```python
from build123d import *

# Parameters (mm, degrees)
F0_W     = 44.45
F0_H     = 44.45
F1_DEPTH = 565.15
F3_DEPTH = 44.45
F5_DEPTH = 44.451
F6_W     = 19.05
F6_H     = 19.05
F7_DEPTH = 19.05


with BuildPart() as f1:
    # F0 (on Top) → F1 (new body)
    with BuildSketch(Plane.XY):
        with Locations((-22.225, 22.225)):
            Rectangle(F0_W, F0_H)
    extrude(amount=-F1_DEPTH)

    # F2 (on face) → F3 (cut, through all)
    with BuildSketch(Plane.XZ):
        Polygon((-9.525, -565.15), (0, -565.15), (0, -488.95), align=None)
    extrude(amount=-F3_DEPTH, mode=Mode.SUBTRACT)

    # F4 (on face) → F5 (cut, through all)
    with BuildSketch(Plane(origin=(-44.45, 0, 0), x_dir=(0, -1, 0), z_dir=(-1, 0, 0))):
        Polygon((0, -565.15), (0, -488.95), (-9.525, -565.15), align=None)
    extrude(amount=-F5_DEPTH, mode=Mode.SUBTRACT)

    # F6 (on face) → F7 (cut)
    with BuildSketch(Plane.XZ):
        with Locations((-9.525, -454.025)):
            Rectangle(F6_W, F6_H)
    extrude(amount=-F7_DEPTH, mode=Mode.SUBTRACT)


solid = f1.part
```
The listing builds one solid part. Answer for the finished solid, in the listing's coordinates (mm). A direction names the side the tool comes from. Give positions to 0.01 mm unless a question says otherwise; leave off trailing zeros.
1) For faces 4 (the face through (-22.536, 4.696, -526.517)), 5 (the face through (-10, 19.05, -454)), determine the directions among +Z, -Z, +X, -X, +Y, -Y from which every point of the face is accessible in a straight line to the end or side of a thin tool.
Reported:
face 4: -Z, +X, -X, -Y
face 5: +X, -Y
2) Determine the mould class of faces 1 (the face through (-4.696, 21.914, -526.517)), 2 (the face through (-10, 9, -444.5)), 3 (the face through (-23, 0, -241)) for opening direction Z: pulls with the +Z half, pulls with the -Z half, needs draft (parallel to the pull), parting line crosses it, or undercut.
Reported:
face 1: pulls with the -Z half
face 2: undercut
face 3: needs draft
3) Consider line 1 along Z through (x, y) = (-14, 16.5); line 2 along X through (y, z) = (22, -498.5); line 3 along Y through (x, z) = (-23.5, -499). Determine where each line is inside the solid, lowest interval first.
Reported:
line 1: z = -565.15 to -463.55, -444.5 to 0
line 2: x = -44.45 to -1.19
line 3: y = 1.26 to 44.45
4) Given P1, Ø9.5, axis at y = 9.5, z = -457.5, coming from the +X side, flat-ended and moving along its own axis, determine where the tip first touches the part or whether it passes through.
Reported:
P1: stops at x = -19.05
